from build123d import *

# Parameters (mm, degrees)
F1_DEPTH = 300
F3_D     = 60
F6_D     = 60
F7_D     = 60


with BuildPart() as f1:
    # F0 (on Front) → F1 (new body)
    with BuildSketch(Plane.XZ):
        Polygon((0, 300), (0, 0), (900, 0), (900, 900), (600, 900), (600, 600), (300, 600), (300, 300), align=None)
    extrude(amount=F1_DEPTH)

    # F3 (through all)
    with Locations(Plane.XY.offset(900)):
        with Locations((750, -150)):
            Hole(F3_D / 2)

    # F6 (through all)
    with Locations(Plane.XY.offset(300)):
        with Locations((150, -150)):
            Hole(F6_D / 2)

    # F7 (through all)
    with Locations(Plane.XY.offset(600)):
        with Locations((450, -150)):
            Hole(F7_D / 2)


solid = f1.part
Source: CAD feature listing. Evaluate the final solid. Frame: model axes, mm. A direction names the side the tool comes from. Round coordinates to 2 decimals unless told otherwise and drop trailing zeros. Loops run counter-clockwise (first coordinate to the right, second up) from the corner with the lowest first, then second, coordinate; pieces in that order, holes last. Notation, with made-up numbers: M 9,83.25 L 45,83.25 A33 cw 45,115.25 Z; hole C 64.25,46 d5. An arc over 180 degrees is marked long. Answer as CSV lines item,"result".
Q1. Cut plane A-A (x = 750). Return the cut outline in (y, z), plus the area to 3 significant figures.
Verdict:
outline,"M -300,0 L -180,0 L -180,900 L -300,900 Z; M -120,0 L 0,0 L 0,900 L -120,900 Z"
area,"216,000 mm^2"
Q2. Cut plane D-D (z = 381). Return the cut outline in (x, y).
Verdict:
outline,"M 300,-300 L 900,-300 L 900,0 L 300,0 Z; hole C 450,-150 d60; hole C 750,-150 d60"
Q3. Cut plane C-C (z = 157). Return the cut outline in (x, y).
Verdict:
outline,"M 0,-300 L 900,-300 L 900,0 L 0,0 Z; hole C 150,-150 d60; hole C 450,-150 d60; hole C 750,-150 d60"
Q4. Line query: line 1 along Y through (x, z) = (150, 96); line 2 along X through (y, z) = (-150.5, 861); line 3 along X through (y, z) = (-130, 467). Output: solid intervals per line, ascending.
Verdict:
line 1,"y = -300 to -180, -120 to 0"
line 2,"x = 600 to 720, 780 to 900"
line 3,"x = 300 to 427.64, 472.36 to 727.64, 772.36 to 900"
Q5. Reachability of faces 4 (the face through (600, -148, 752)), 5 (the face through (156.503, -179.287, 147.9)) from +Z, -Z, +X, -X, +Y, -Y: full face, straight path, thin tool, end or side. Return the list, or none.
Verdict:
face 4,"+Z, -X, +Y, -Y"
face 5,"+Z, -Z"
Q6. Cut plane B-B (y = -150). Return the cut outline in (x, z), plus the area to 3 significant figures.
Verdict:
outline,"M 0,0 L 120,0 L 120,300 L 0,300 Z; M 180,0 L 420,0 L 420,600 L 300,600 L 300,300 L 180,300 Z; M 480,0 L 720,0 L 720,900 L 600,900 L 600,600 L 480,600 Z; M 780,0 L 900,0 L 900,900 L 780,900 Z"
area,"432,000 mm^2"
Q7. Contact query for a flat-ended pin moving along its axis: pin 1 (1.5 mm diameter, centred on y = -63.5, z = 488, fed in from -X). Output: stop coordinate, or through.
Verdict:
pin 1,"stops at x = 300"
Q8. Pull-direction query (X, two-part tool) for faces 1 (the face through (422.288, -161.49, 295.8)), 2 (the face through (300, -148, 452)), 3 (the face through (485, -148, 600)); classes: +X half, -X half, draft (parallel to the pull), parting line (faces both ways), or undercut.
Verdict:
face 1,"undercut"
face 2,"-X half"
face 3,"draft"
